Autodesk Inventor part; units mm, degrees
ref_plane "YZ Plane" through (0, 0, 0) normal (1, 0, 0) x (0, 1, 0)
ref_plane "XZ Plane" through (0, 0, 0) normal (0, 1, 0) x (-1, 0, 0)
ref_plane "XY Plane" through (0, 0, 0) normal (0, 0, 1) x (1, 0, 0)
sketch "Sketch1" plane through (0, 0, 0) normal (0, 0, 1) x (1, 0, 0)
  line L0 (-31, 44) -> (-31, 55.9)
  line L1 (-31, 55.9) -> (-37.25, 55.9)
  line L2 (-37.25, 55.9) -> (-37.25, 62.1)
  line L3 (-37.25, 62.1) -> (-31, 62.1)
  line L4 (-31, 62.1) -> (-31, 64)
  line L5 (-31, 64) -> (-25, 64)
  line L6 (-25, 64) -> (-25, 67)
  arc A0 (-23, 69) -> (-25, 67) centre (-23, 67) ccw
  line L7 (-23, 69) -> (-17, 69)
  arc A1 (-15, 67) -> (-17, 69) centre (-17, 67) ccw
  line L8 (-15, 67) -> (-15, 64)
  line L9 (-15, 64) -> (-6, 64)
  line L10 (-6, 64) -> (-6, 44)
  line L11 (-6, 44) -> (-31, 44)
  line L12 (-61.6, 39.5) -> (-61.6, 60.5)
  line L13 (-61.6, 60.5) -> (-46.4, 60.5)
  line L14 (-46.4, 60.5) -> (-46.4, 39.5)
  line L15 (-46.4, 39.5) -> (-61.6, 39.5)
  circle A2 centre (-30.9, 77.8) radius 3
  circle A3 centre (-3, 59) radius 1.5
  circle A4 centre (-26.5, 18.5) radius 1.5
  circle A5 centre (-26.5, 4.5) radius 1.5
  circle A6 centre (-55.5, 4.5) radius 1.5
  circle A7 centre (-55.5, 18.5) radius 1.5
  circle A8 centre (-3, 19.5) radius 1.5
  circle A9 centre (-9.5, 19.5) radius 1.5
  circle A10 centre (-60.5, 68.5) radius 1.5
  circle A11 centre (-60.5, 82.5) radius 1.5
  circle A12 centre (-2.5, 82.5) radius 1.5
  circle A13 centre (-2.5, 68.5) radius 1.5
  arc A14 (0, 83) -> (-4, 87) centre (-4, 83) ccw
  line L16 (-4, 87) -> (-59, 87)
  arc A15 (-59, 87) -> (-63, 83) centre (-59, 83) ccw
  line L17 (-63, 83) -> (-63, 26.3448)
  arc A16 (-63, 26.3448) -> (-60.5004, 22.6368) centre (-59, 26.3448) ccw
  arc A17 (-58.0008, 18.9289) -> (-60.5004, 22.6368) centre (-62.0008, 18.9289) ccw
  line L18 (-58.0008, 18.9289) -> (-58.0008, 4)
  arc A18 (-58.0008, 4) -> (-54.0008, 0) centre (-54.0008, 4) ccw
  line L19 (-54.0008, 0) -> (-24, 0)
  line L20 (-24, 0) -> (-24, 6.4)
  line L21 (-24, 6.4) -> (-21, 6.4)
  line L22 (-21, 6.4) -> (-21, 33.4)
  line L23 (-21, 33.4) -> (-15, 33.4)
  line L24 (-15, 33.4) -> (-15, 6.4)
  line L25 (-15, 6.4) -> (-9, 6.4)
  line L26 (-9, 6.4) -> (-9, 13.4)
  line L27 (-9, 13.4) -> (-10.25, 13.4)
  line L28 (-10.25, 13.4) -> (-10.25, 15.2)
  line L29 (-10.25, 15.2) -> (-9, 15.2)
  line L30 (-9, 15.2) -> (-9, 17)
  line L31 (-9, 17) -> (-6, 17)
  line L32 (-6, 17) -> (-6, 15.2)
  line L33 (-6, 15.2) -> (-4.75, 15.2)
  line L34 (-4.75, 15.2) -> (-4.75, 13.4)
  line L35 (-4.75, 13.4) -> (-6, 13.4)
  line L36 (-6, 13.4) -> (-6, 6.4)
  line L37 (-6, 6.4) -> (0, 6.4)
  line L38 (0, 6.4) -> (0, 83)
  point P0 (0, 0)
  point P1 (0, 0)
extrude "Extrusion1" add sketch "Sketch1" along normal blind 6
properties part number "yCarTop"
Read the model definition and answer for the solid it produces. Units are mm, in the model's axes. A direction names the side the tool comes from. Round coordinates to 2 decimals unless told otherwise and drop trailing zeros. Order: outer loops, then holes, each group sorted by start corner. A loop starts at its lowest first (then second) coordinate and runs counter-clockwise, first axis right, second up. Notation, with made-up numbers: (44.25, -24.5) - (72.25, -24.5) arc R24 ccw to (72.25, -9.5) - close; hole circle Ø7 at (-8.75, -4). An arc over 180 degrees is marked (long way). Use one line per item in the form item = value. Start each with the question number.
(1) The part is cut by section D-D (x = -26.5). Give the vertices of the cut face in (y, z), then the cut area to 3 significant figures.
(2) The part is cut by section A-A (y = 59). Give the vertices of the cut face in (x, z).
(3) The part is cut by section C-C (y = 42.5). Give the vertices of the cut face in (x, z), then the cut area to 3 significant figures.
(4) For faces 4 (the face through (-15, 20, 3)), 5 (the face through (-58.001, 12, 3)), 6 (the face through (-46.4, 50, 3)), 7 (the face through (-3, 6.4, 3)), determine the directions among +Z, -Z, +X, -X, +Y, -Y from which every point of the face is accessible in a straight line to the end or side of a thin tool.
(5) Determine the mould class of faces 1 (the face through (-31, 87, 3)), 2 (the face through (-24, 3, 3)), 3 (the face through (-18, 33.4, 3)) for opening direction X: +X half, -X half, draft (parallel to the pull), parting line (faces both ways), or undercut.
(6) Find the intervals of material crossed by line 1 along X through (y, z) = (82.5, 3.6); line 2 along X through (y, z) = (13, 5.45); line 3 along Y through (x, z) = (-30.9, 2.3), in increasing order. Write a range as from..to.
(7) Flat-ended cylindrical pins translate along their axes: pin 1 Ø1.8 at (y, z) = (15, 3.5) entering from -X; pin 2 Ø1.8 at (x, y) = (-60.5, 68.5) entering from -Z; pin 3 Ø1 at (y, z) = (22, 4) entering from -X; pin 4 Ø3 at (x, z) = (-20, 2) entering from -Y. Find the tip coordinate at first contact, or state that the pin passes through.
(8) The part is cut by section B-B (x = -19). Give the vertices of the cut face in (y, z), then the cut area to 3 significant figures.
Checked values:
q1.outline = (0, 0) - (3, 0) - (3, 6) - (0, 6) - close; (6, 0) - (17, 0) - (17, 6) - (6, 6) - close; (20, 0) - (44, 0) - (44, 6) - (20, 6) - close; (64, 0) - (87, 0) - (87, 6) - (64, 6) - close
q1.area = 366 mm^2
q2.outline = (-63, 0) - (-61.6, 0) - (-61.6, 6) - (-63, 6) - close; (-46.4, 0) - (-37.25, 0) - (-37.25, 6) - (-46.4, 6) - close; (-6, 0) - (-4.5, 0) - (-4.5, 6) - (-6, 6) - close; (-1.5, 0) - (0, 0) - (0, 6) - (-1.5, 6) - close
q3.outline = (-63, 0) - (-61.6, 0) - (-61.6, 6) - (-63, 6) - close; (-46.4, 0) - (0, 0) - (0, 6) - (-46.4, 6) - close
q3.area = 287 mm^2
q4.face_4 = +Z, -Z, -Y
q4.face_5 = +Z, -Z, -X, -Y
q4.face_6 = +Z, -Z
q4.face_7 = +Z, -Z, +X, -Y
q5.face_1 = draft
q5.face_2 = +X half
q5.face_3 = undercut
q6.line_1 = -63..-62, -59..-4, -1..0
q6.line_2 = -58..-21, -15..-9, -6..0
q6.line_3 = 0..44, 64..74.8, 80.8..87
q7.pin_1 = -58
q7.pin_2 = through
q7.pin_3 = -60.2
q7.pin_4 = 6.4
q8.outline = (33.4, 0) - (44, 0) - (44, 6) - (33.4, 6) - close; (69, 0) - (87, 0) - (87, 6) - (69, 6) - close
q8.area = 172 mm^2
